For this review, take the finished solid that the model builds, in its own axes (mm). Give positions to 0.01 mm unless a question says otherwise; leave off trailing zeros. Write each loop counter-clockwise with the first axis right and the second up, starting at its lowest first coordinate (ties: lowest second). Pieces come first, ordered by that corner, then holes. Notation, with made-up numbers: (33, 57.25) -> (37, 57.25) arc R29 ccw to (37, 79.25) -> close; hole circle Ø3 at (70, 24.5). An arc over 180 degrees is marked (long way). Answer as CSV lines item,"result".
Autodesk Fusion 360 part; units mm, degrees
sketch "plate-2025-12-07T05_26_02.564Z" plane through (0, 0, 0) normal (0, 0, 1) x (1, 0, 0)
  line L0 (3.025, -2.525) -> (16.025, -2.525)
  line L1 (3.025, -16.525) -> (16.025, -16.525)
  line L2 (2.525, -3.025) -> (2.525, -16.025)
  line L3 (16.525, -3.025) -> (16.525, -16.025)
  arc A0 (3.025, -2.525) -> (2.525, -3.025) centre (3.025, -3.025) ccw
  arc A1 (16.525, -3.025) -> (16.025, -2.525) centre (16.025, -3.025) ccw
  arc A2 (2.525, -16.025) -> (3.025, -16.525) centre (3.025, -16.025) ccw
  arc A3 (16.025, -16.525) -> (16.525, -16.025) centre (16.025, -16.025) ccw
  line L4 (41.125, -2.525) -> (54.125, -2.525)
  line L5 (41.125, -16.525) -> (54.125, -16.525)
  line L6 (40.625, -3.025) -> (40.625, -16.025)
  line L7 (54.625, -3.025) -> (54.625, -16.025)
  arc A4 (41.125, -2.525) -> (40.625, -3.025) centre (41.125, -3.025) ccw
  arc A5 (54.625, -3.025) -> (54.125, -2.525) centre (54.125, -3.025) ccw
  arc A6 (40.625, -16.025) -> (41.125, -16.525) centre (41.125, -16.025) ccw
  arc A7 (54.125, -16.525) -> (54.625, -16.025) centre (54.125, -16.025) ccw
  line L8 (3.025, -21.575) -> (16.025, -21.575)
  line L9 (3.025, -35.575) -> (16.025, -35.575)
  line L10 (2.525, -22.075) -> (2.525, -35.075)
  line L11 (16.525, -22.075) -> (16.525, -35.075)
  arc A8 (3.025, -21.575) -> (2.525, -22.075) centre (3.025, -22.075) ccw
  arc A9 (16.525, -22.075) -> (16.025, -21.575) centre (16.025, -22.075) ccw
  arc A10 (2.525, -35.075) -> (3.025, -35.575) centre (3.025, -35.075) ccw
  arc A11 (16.025, -35.575) -> (16.525, -35.075) centre (16.025, -35.075) ccw
  line L12 (22.075, -21.575) -> (35.075, -21.575)
  line L13 (22.075, -35.575) -> (35.075, -35.575)
  line L14 (21.575, -22.075) -> (21.575, -35.075)
  line L15 (35.575, -22.075) -> (35.575, -35.075)
  arc A12 (22.075, -21.575) -> (21.575, -22.075) centre (22.075, -22.075) ccw
  arc A13 (35.575, -22.075) -> (35.075, -21.575) centre (35.075, -22.075) ccw
  arc A14 (21.575, -35.075) -> (22.075, -35.575) centre (22.075, -35.075) ccw
  arc A15 (35.075, -35.575) -> (35.575, -35.075) centre (35.075, -35.075) ccw
  line L16 (41.125, -21.575) -> (54.125, -21.575)
  line L17 (41.125, -35.575) -> (54.125, -35.575)
  line L18 (40.625, -22.075) -> (40.625, -35.075)
  line L19 (54.625, -22.075) -> (54.625, -35.075)
  arc A16 (41.125, -21.575) -> (40.625, -22.075) centre (41.125, -22.075) ccw
  arc A17 (54.625, -22.075) -> (54.125, -21.575) centre (54.125, -22.075) ccw
  arc A18 (40.625, -35.075) -> (41.125, -35.575) centre (41.125, -35.075) ccw
  arc A19 (54.125, -35.575) -> (54.625, -35.075) centre (54.125, -35.075) ccw
  line L20 (12.55, -40.625) -> (25.55, -40.625)
  line L21 (12.55, -54.625) -> (25.55, -54.625)
  line L22 (12.05, -41.125) -> (12.05, -54.125)
  line L23 (26.05, -41.125) -> (26.05, -54.125)
  arc A20 (12.55, -40.625) -> (12.05, -41.125) centre (12.55, -41.125) ccw
  arc A21 (26.05, -41.125) -> (25.55, -40.625) centre (25.55, -41.125) ccw
  arc A22 (12.05, -54.125) -> (12.55, -54.625) centre (12.55, -54.125) ccw
  arc A23 (25.55, -54.625) -> (26.05, -54.125) centre (25.55, -54.125) ccw
  line L24 (31.6, -40.625) -> (44.6, -40.625)
  line L25 (31.6, -54.625) -> (44.6, -54.625)
  line L26 (31.1, -41.125) -> (31.1, -54.125)
  line L27 (45.1, -41.125) -> (45.1, -54.125)
  arc A24 (31.6, -40.625) -> (31.1, -41.125) centre (31.6, -41.125) ccw
  arc A25 (45.1, -41.125) -> (44.6, -40.625) centre (44.6, -41.125) ccw
  arc A26 (31.1, -54.125) -> (31.6, -54.625) centre (31.6, -54.125) ccw
  arc A27 (44.6, -54.625) -> (45.1, -54.125) centre (44.6, -54.125) ccw
  line L28 (-11.896, 34.298) -> (70.017, 34.298)
  line L29 (70.017, 34.298) -> (70.017, -69.046)
  line L30 (70.017, -69.046) -> (-11.896, -69.046)
  line L31 (-11.896, -69.046) -> (-11.896, 34.298)
  line L32 (20.315, 34.298) -> (38.815, 34.298)
  line L33 (38.815, 34.298) -> (38.815, 3.298)
  line L34 (38.815, 3.298) -> (20.315, 3.298)
  line L35 (20.315, 3.298) -> (20.315, 34.298)
  circle A28 centre (-6.896, 29.298) radius 1.7
  circle A29 centre (65.017, 29.298) radius 1.7
  circle A30 centre (-6.896, -64.046) radius 1.7
  circle A31 centre (65.017, -64.046) radius 1.7
  dimension "d1" = 81.913
  dimension "d2" = 103.344
  dimension "d3" = 23.946
  dimension "d4" = 14.421
  dimension "d5" = 18.5
  dimension "d6" = 31
  dimension "d7" = 32.211
  dimension "d8" = 3.4
  dimension "d9" = 3.4
  dimension "d10" = 3.4
  dimension "d11" = 3.4
  dimension "d12" = 5
  dimension "d13" = 5
  dimension "d14" = 5
  dimension "d15" = 5
  dimension "d16" = 5
  dimension "d17" = 5
  dimension "d18" = 5
  dimension "d19" = 5
extrude "Extrude1" add sketch "plate-2025-12-07T05_26_02.564Z" along normal blind 1.5 contours L28 L29 L30 L31 L33 L34 L35
fillet "Fillet1" radius 5 4 edges at (-11.896, -69.046, 0.75) (70.017, -69.046, 0.75) (70.017, 34.298, 0.75) (-11.896, 34.298, 0.75)
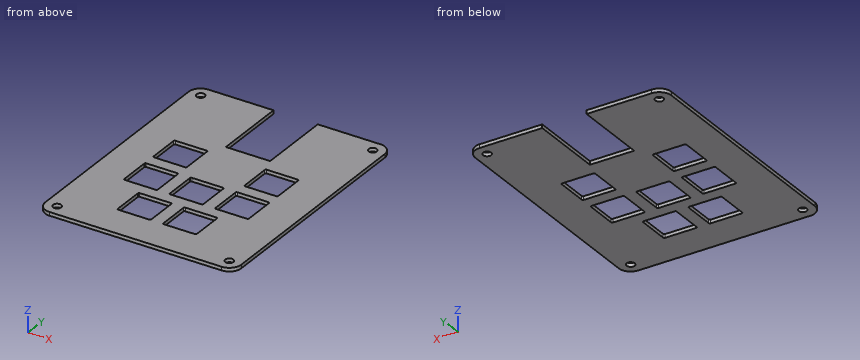
Q1. To check wall thickness, follow probe 1 along X at (y, z) = (-45.5, 0.65); probe 2 along X at (y, z) = (-14, 0.7) (3 decimals); probe 3 along X at (y, z) = (-26.5, 1.4) (3 decimals). State the ranges of each line that lie inside material, in increasing order. Write a range as [from, to].
Answer block:
probe 1,"x = [-11.9, 12.05], [26.05, 31.1], [45.1, 70.02]"
probe 2,"x = [-11.896, 2.525], [16.525, 40.625], [54.625, 70.017]"
probe 3,"x = [-11.896, 2.525], [16.525, 21.575], [35.575, 40.625], [54.625, 70.017]"
Q2. Clearance check with a flat-ended pin moving along its axis: pin 1 (5.5 mm diameter, centred on x = 65.017, y = -64.046, fed in from +Z). State where the tip first meets the part, or that it passes through.
Answer block:
pin 1,"stops at z = 1.5"
Q3. Add section D-D (y = -30.5). Write out the cut boundary in (x, z) (3 decimals), plus the area to 3 significant figures.
Answer block:
outline,"(-11.896, 0) -> (2.525, 0) -> (2.525, 1.5) -> (-11.896, 1.5) -> close; (16.525, 0) -> (21.575, 0) -> (21.575, 1.5) -> (16.525, 1.5) -> close; (35.575, 0) -> (40.625, 0) -> (40.625, 1.5) -> (35.575, 1.5) -> close; (54.625, 0) -> (70.017, 0) -> (70.017, 1.5) -> (54.625, 1.5) -> close"
area,"59.9 mm2"
Q4. Add section C-C (x = 29.5). Write out the cut boundary in (y, z) (3 decimals).
Answer block:
outline,"(-69.046, 0) -> (-35.575, 0) -> (-35.575, 1.5) -> (-69.046, 1.5) -> close; (-21.575, 0) -> (3.298, 0) -> (3.298, 1.5) -> (-21.575, 1.5) -> close"
Q5. Add section B-B (x = 49). Write out the cut boundary in (y, z) (3 decimals), plus the area to 3 significant figures.
Answer block:
outline,"(-69.046, 0) -> (-35.575, 0) -> (-35.575, 1.5) -> (-69.046, 1.5) -> close; (-21.575, 0) -> (-16.525, 0) -> (-16.525, 1.5) -> (-21.575, 1.5) -> close; (-2.525, 0) -> (34.298, 0) -> (34.298, 1.5) -> (-2.525, 1.5) -> close"
area,"113 mm2"
Q6. Add section A-A (y = 5.5). Write out the cut boundary in (x, z) (3 decimals).
Answer block:
outline,"(-11.896, 0) -> (20.315, 0) -> (20.315, 1.5) -> (-11.896, 1.5) -> close; (38.815, 0) -> (70.017, 0) -> (70.017, 1.5) -> (38.815, 1.5) -> close"
